Work out the finished part from the listing and answer in its coordinate system (mm). Face numbers are marked on the shaded views. Give positions to 0.01 mm unless a question says otherwise; leave off trailing zeros. Order: outer loops, then holes, each group sorted by start corner. A loop starts at its lowest first (then second) coordinate and runs counter-clockwise, first axis right, second up. Notation, with made-up numbers: (89.25, 44.25) -> (127.25, 44.25) arc R30 ccw to (127.25, 72.25) -> close; hole circle Ø11 at (-27.5, 70.25). An arc over 180 degrees is marked (long way). Answer as CSV lines item,"result". Start each with the question number.
1. For a pull along Y with two mould halves and no side action, classify the marked faces 1, 2 and 3 as released by +Y, released by -Y, zero draft, split by the parting line, or undercut.
2. A cutting plane is placed at C-C (z = 29). Give the vertices of the cut face in (x, y).
3. A cutting plane is placed at A-A (x = 3.75). Give the vertices of the cut face in (y, z), then the cut area to 3 significant figures.
4. Flat-ended cylindrical pins translate along their axes: pin 1 (0.6 mm diameter, centred on x = 11, y = 0.5, fed in from -Z); pin 2 (0.9 mm diameter, centred on x = 11, z = 9.5, fed in from +Y); pin 3 (4 mm diameter, centred on x = 9, y = 21.5, fed in from +Z); pin 4 (2 mm diameter, centred on x = 8.5, z = 39, fed in from -Y). Find the tip coordinate at first contact, or state that the pin passes through.
5. A cutting plane is placed at B-B (y = 18). Give the vertices of the cut face in (x, z).
6. Find the intervals of material crossed by L1, parallel to X at y = 30.5, z = 29; L2, parallel to Y at x = 4.5, z = 0.5; L3, parallel to Y at x = 9, z = -7.5, in increasing order.
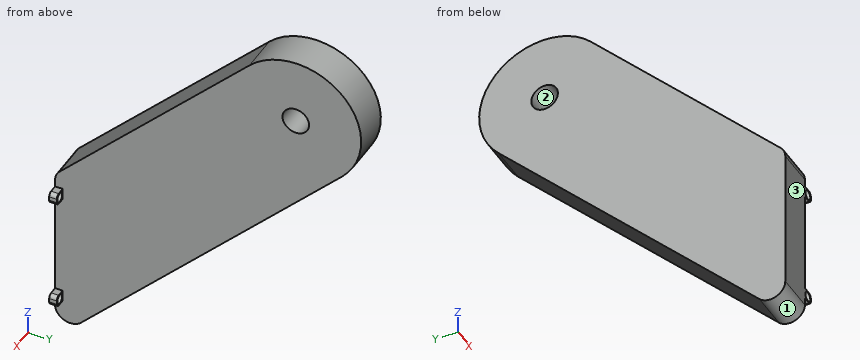
from build123d import *

# Parameters (mm, degrees)
SKETCH1_R           = 3.5
BOSS_EXTRUDE2_DEPTH = 10
SKETCH2_W           = 3
SKETCH2_H           = 3
SKETCH2_R           = 1.25
BOSS_EXTRUDE3_DEPTH = 2
FILLET2_R           = 1
FILLET6_R           = 1
FILLET7_R           = 1


with BuildPart() as part:
    # Sketch1 → Boss-Extrude2 (new body)
    with BuildSketch(Plane(origin=(0, 0, 0), x_dir=(0, 0, -1), z_dir=(1, 0, 0))):
        with BuildLine():
            Line((0, 0), (-13.343145751, 0))
            ThreePointArc((-13.343145751, 0), (-14.87387948, 0.30448187), (-16.171572875, 1.171572875))
            Line((-16.171572875, 1.171572875), (-66.154328925, 51.154328925))
            ThreePointArc((-66.154328925, 51.154328925), (-66.154328925, 75.497474674), (-41.811183175, 75.497474674))
            Line((-41.811183175, 75.497474674), (26.857864374, 6.828427125))
            ThreePointArc((26.857864374, 6.828427125), (27.72495538, 2.469266271), (24.029437249, 0))
            Line((24.029437249, 0), (0, 0))
        make_face()
        with Locations((-53.98275605, 63.3259018)):
            Circle(SKETCH1_R, mode=Mode.SUBTRACT)
    extrude(amount=BOSS_EXTRUDE2_DEPTH)

    # Sketch2 → Boss-Extrude3 (add)
    # profile 1 of 2: a face of its own
    with BuildSketch(Plane.XZ):
        with Locations((11.5, 9.843145751)):
            Rectangle(SKETCH2_W, SKETCH2_H)
        with Locations(Location((11.5, 9.843145751, 0), (0, 0, 270))):
            Circle(SKETCH2_R, mode=Mode.SUBTRACT)
    # profile 2 of 2: a face of its own
    with BuildSketch(Plane.XZ):
        with Locations((11.5, -20.529437249)):
            Rectangle(SKETCH2_W, SKETCH2_H)
        with Locations(Location((11.5, -20.529437249, 0), (0, 0, 270))):
            Circle(SKETCH2_R, mode=Mode.SUBTRACT)
    extrude(amount=-BOSS_EXTRUDE3_DEPTH)

    # Fillet2
    fillet2_edges = [part.edges().sort_by_distance(p)[0] for p in [
        (13, 1, 11.343145751),
    ]]
    fillet(fillet2_edges, radius=FILLET2_R)

    # Fillet6
    fillet6_edges = [part.edges().sort_by_distance(p)[0] for p in [
        (13, 1, 8.343145751),
    ]]
    fillet(fillet6_edges, radius=FILLET6_R)

    # Fillet7
    fillet7_edges = [part.edges().sort_by_distance(p)[0] for p in [
        (13, 1, -19.029437249),
        (13, 1, -22.029437249),
    ]]
    fillet(fillet7_edges, radius=FILLET7_R)


solid = part.part
Answer sheet:
1,face 1,"split by the parting line"
1,face 2,"undercut"
1,face 3,"released by -Y"
2,outline,"(0, 14) -> (10, 14) -> (10, 62.69) -> (0, 62.69) -> close"
3,outline,"(0, -24.03) arc R4 ccw to (6.83, -26.86) -> (75.5, 41.81) arc R17.21 ccw to (51.15, 66.15) -> (1.17, 16.17) arc R4 ccw to (0, 13.34) -> close; hole circle Ø7 at (63.33, 53.98)"
3,area,"3,490 mm^2"
4,pin 1,"stops at z = -22.03"
4,pin 2,"passes through"
4,pin 3,"stops at z = 38.5"
4,pin 4,"stops at y = 23"
5,outline,"(0, -15.69) -> (10, -15.69) -> (10, 33) -> (0, 33) -> close"
6,L1,"x = 0 to 10"
6,L2,"y = 0 to 34.19"
6,L3,"y = 0 to 26.19"
